Autodesk Inventor part; units mm, degrees
ref_plane "YZ Plane" through (0, 0, 0) normal (1, 0, 0) x (0, 1, 0)
ref_plane "XZ Plane" through (0, 0, 0) normal (0, 1, 0) x (-1, 0, 0)
ref_plane "XY Plane" through (0, 0, 0) normal (0, 0, 1) x (1, 0, 0)
sketch "Sketch1" plane through (0, 0, 0) normal (0, 0, 1) x (1, 0, 0)
  line L0 (83.5624, -61.7466) -> (89.5624, -61.7716)
  line L1 (89.5624, -61.7716) -> (94.5924, -64.7466)
  line L2 (94.5924, -64.7466) -> (94.5924, -114.4666)
  line L3 (94.5924, -114.4666) -> (142.9124, -114.4666)
  line L4 (142.9124, -114.4666) -> (142.9124, -64.7466)
  line L5 (142.9124, -64.7466) -> (148.0124, -61.7466)
  line L6 (148.0124, -61.7466) -> (153.9624, -61.7466)
  arc A0 (153.9624, -61.7466) -> (83.5624, -61.7466) centre (118.7624, -61.7466) ccw
  line L7 (96.775, -95.75) -> (96.775, -78.75)
  line L8 (96.775, -78.75) -> (116.275, -78.75)
  line L9 (116.275, -78.75) -> (116.275, -95.75)
  line L10 (116.275, -95.75) -> (96.775, -95.75)
  line L11 (121.25, -95.775) -> (121.25, -78.775)
  line L12 (121.25, -78.775) -> (140.75, -78.775)
  line L13 (140.75, -78.775) -> (140.75, -95.775)
  line L14 (140.75, -95.775) -> (121.25, -95.775)
  line L15 (130.3424, -108.4516) -> (130.6424, -108.4516)
  arc A1 (130.6424, -109.0016) -> (130.6424, -108.4516) centre (130.6424, -108.7266) ccw
  line L16 (130.6424, -109.0016) -> (130.3424, -109.0016)
  arc A2 (130.3424, -108.4516) -> (130.3424, -109.0016) centre (130.3424, -108.7266) ccw
  line L17 (135.3424, -108.4516) -> (135.6424, -108.4516)
  arc A3 (135.6424, -109.0016) -> (135.6424, -108.4516) centre (135.6424, -108.7266) ccw
  line L18 (135.6424, -109.0016) -> (135.3424, -109.0016)
  arc A4 (135.3424, -108.4516) -> (135.3424, -109.0016) centre (135.3424, -108.7266) ccw
  line L19 (129.7424, -111.1016) -> (129.7424, -111.7516)
  arc A5 (129.2424, -111.7516) -> (129.7424, -111.7516) centre (129.4924, -111.7516) ccw
  line L20 (129.2424, -111.7516) -> (129.2424, -111.1016)
  arc A6 (129.7424, -111.1016) -> (129.2424, -111.1016) centre (129.4924, -111.1016) ccw
  line L21 (136.7424, -111.1016) -> (136.7424, -111.7516)
  arc A7 (136.2424, -111.7516) -> (136.7424, -111.7516) centre (136.4924, -111.7516) ccw
  line L22 (136.2424, -111.7516) -> (136.2424, -111.1016)
  arc A8 (136.7424, -111.1016) -> (136.2424, -111.1016) centre (136.4924, -111.1016) ccw
  circle A9 centre (88.0524, -59.1866) radius 0.45
  circle A10 centre (85.5195, -59.3771) radius 0.45
  circle A11 centre (112.8524, -37.2166) radius 0.45
  circle A12 centre (110.6984, -38.5626) radius 0.45
  circle A13 centre (127.4524, -38.4866) radius 0.45
  circle A14 centre (125.2984, -37.1406) radius 0.45
  circle A15 centre (129.9924, -44.7466) radius 0.45
  circle A16 centre (128.5355, -42.666) radius 0.45
  circle A17 centre (146.5124, -56.2766) radius 0.45
  circle A18 centre (143.9833, -56.042) radius 0.45
  circle A19 centre (117.3124, -33.4566) radius 0.45
  circle A20 centre (115.1584, -34.8026) radius 0.45
  circle A21 centre (105.3925, -47.0869) radius 0.45
  circle A22 centre (103.8924, -49.1366) radius 0.45
  circle A23 centre (133.2993, -49.4472) radius 0.45
  circle A24 centre (131.8424, -47.3666) radius 0.45
  circle A25 centre (122.9924, -34.4966) radius 0.45
  circle A26 centre (120.8384, -33.1506) radius 0.45
  circle A27 centre (151.7915, -59.8612) radius 0.45
  circle A28 centre (149.2624, -59.6266) radius 0.45
  circle A29 centre (93.5153, -55.9661) radius 0.45
  circle A30 centre (90.9824, -56.1566) radius 0.45
  circle A31 centre (108.6624, -42.1366) radius 0.45
  circle A32 centre (107.1623, -44.1863) radius 0.45
  circle A33 centre (25.5324, -58.5866) radius 0.5
  circle A34 centre (22.9924, -58.5866) radius 0.5
  circle A35 centre (20.4524, -58.5866) radius 0.5
  circle A36 centre (17.9124, -58.5866) radius 0.5
  circle A37 centre (108.7824, -100.5166) radius 0.5
  circle A38 centre (108.7824, -97.9766) radius 0.5
  circle A39 centre (106.2424, -100.5166) radius 0.5
  circle A40 centre (106.2424, -97.9766) radius 0.5
  circle A41 centre (103.7024, -100.5166) radius 0.5
  circle A42 centre (103.7024, -97.9766) radius 0.5
  circle A43 centre (97.2624, -105.2666) radius 1
  circle A44 centre (97.2624, -69.2666) radius 1
  circle A45 centre (117.6824, -75.6166) radius 0.45
  circle A46 centre (120.1824, -75.6166) radius 0.45
  circle A47 centre (121.7624, -124.4716) radius 0.381
  circle A48 centre (118.7624, -124.4716) radius 0.381
  circle A49 centre (115.7624, -124.4716) radius 0.381
  circle A50 centre (140.2874, -69.2666) radius 1
  circle A51 centre (140.2874, -105.2666) radius 1
  circle A52 centre (129.0424, -98.2966) radius 0.5
  circle A53 centre (129.0424, -100.8366) radius 0.5
  circle A54 centre (131.5824, -98.2966) radius 0.5
  circle A55 centre (131.5824, -100.8366) radius 0.5
  circle A56 centre (134.1224, -98.2966) radius 0.5
  circle A57 centre (134.1224, -100.8366) radius 0.5
extrude "Micromouse1.2.kicad_pcb_Outline" add sketch "Sketch1" along normal blind 1.6
sketch "Sketch2" plane through (25.5324, -58.5866, 1.6) normal (0, 0, 1) x (1, 0, 0)
  circle A0 centre (-7.62, 0) radius 0.5
  circle A1 centre (-5.08, 0) radius 0.5
  circle A2 centre (-2.54, 0) radius 0.5
  circle A3 centre (0, 0) radius 0.5
  circle A4 centre (90.23, -65.885) radius 0.381
  circle A5 centre (93.23, -65.885) radius 0.381
  circle A6 centre (96.23, -65.885) radius 0.381
  point P0 (-25.5324, 58.5866)
extrude "Extrusion2" cut sketch "Sketch2" against normal through all
properties part number "Micromouse1.2.kicad_pcb"
Part model, mm, in its own coordinate system. Coordinates: 2 decimals unless noted, no trailing zeros. Write each loop counter-clockwise with the first axis right and the second up, starting at its lowest first coordinate (ties: lowest second). Pieces come first, ordered by that corner, then holes.
Item 1: Slice it at A-A (x = 138). Write the cut outline in (y, z) (3 decimals), and give its area (3 significant figures).
Item 2: Mould opens along X. For faces 1 (the face through (118, -70, 1.6)), 2 (the face through (145.427, -63.268, 0.789)), 3 (the face through (97.724, -68.379, 0.789)) say: released by +X, released by -X, zero draft, split by the parting line, or undercut.
Item 3: Slice it at B-B (z = 1.1). Count the separate pieces of the cut face and the enclosed holes in it, and give its area (3 significant figures).
Item 4: Slice it at C-C (x = 100.5). Write the cut outline in (y, z), and give its area (3 significant figures).
Item 5: Pin check, flat tips, straight feed: pin 1 (0.7 mm diameter, centred on y = -111.5, z = 0.5, fed in from -X); pin 2 (5 mm diameter, centred on x = 93, y = -81.5, fed in from -Z); pin 3 (0.5 mm diameter, centred on y = -111.5, z = 1, fed in from +X). Stop position of each tip, or through.
Item 6: Probe line 1 (X direction, y = -82.5, z = 1.35) (3 decimals); line 2 (Y direction, x = 88, z = 0.6); line 3 (Y direction, x = 134.5, z = 0.1) (3 decimals). List the from-to ranges inside material, lowest first.
Results found:
1. outline: (-114.467, 0) - (-95.775, 0) - (-95.775, 1.6) - (-114.467, 1.6) - close; (-78.775, 0) - (-32.269, 0) - (-32.269, 1.6) - (-78.775, 1.6) - close
1. area: 104 mm2
2. face 1: zero draft
2. face 2: released by +X
2. face 3: undercut
3. separate pieces: 1
3. enclosed holes: 48
3. area: 3,810 mm2
4. outline: (-114.47, 0) - (-95.75, 0) - (-95.75, 1.6) - (-114.47, 1.6) - close; (-78.75, 0) - (-31.65, 0) - (-31.65, 1.6) - (-78.75, 1.6) - close
4. area: 105 mm2
5. pin 1: stops at x = 94.59
5. pin 2: stops at z = 0
5. pin 3: stops at x = 142.91
6. line 1: x = 94.592 to 96.775, 116.275 to 121.25, 140.75 to 142.912
6. line 2: y = -61.77 to -59.63, -58.74 to -44.64
6. line 3: y = -114.467 to -101.164, -100.509 to -98.624, -97.969 to -95.775, -78.775 to -30.261
